Autodesk Inventor part; units mm, degrees
ref_plane "YZ Plane" through (0, 0, 0) normal (1, 0, 0) x (0, 1, 0)
ref_plane "XZ Plane" through (0, 0, 0) normal (0, 1, 0) x (-1, 0, 0)
ref_plane "XY Plane" through (0, 0, 0) normal (0, 0, 1) x (1, 0, 0)
sketch "Sketch1" plane through (0, 0, 0) normal (0, 1, 0) x (-1, 0, 0)
  line L0 (-22, -5) -> (22, -5)
  line L1 (22, 0) -> (22, 0)
  line L2 (22, 5) -> (-22, 5)
  line L3 (-22, 0) -> (-22, 0)
  line L4 (-22, -5) -> (22, 5) construction
  line L5 (22, -5) -> (-22, 5) construction
  circle A0 centre (19.5, 0) radius 1
  line L6 (-22, 5) -> (-22, -5)
  line L7 (22, 5) -> (22, -5)
  circle A1 centre (-19.5, 0) radius 1
  point P0 (0, 0)
  dimension "d0" = 10
  dimension "d1" = 44
  dimension "d3" = 2
  dimension "d6" = 2.5
  dimension "d8" = 5
  dimension "d13" = 2
  dimension "d14" = 2.5
  dimension "d15" = 5
extrude "Extrusion1" add sketch "Sketch1" along normal blind 5
properties part number "link"
Verification items for the finished model (mm, model axes). Give positions to 0.01 mm unless a question says otherwise; leave off trailing zeros. Loops run counter-clockwise (first coordinate to the right, second up) from the corner with the lowest first, then second, coordinate; pieces in that order, holes last. Notation, with made-up numbers: (-9, 23.25) - (19, 23.25) arc R24 cw to (19, 47.25) - close; hole circle Ø6 at (-33.5, 48). An arc over 180 degrees is marked (long way). Write item = value, one per line. Start each with the question number.
Q1. Cross-section at B-B, the plane z = 0. Enter the section's corners in (x, y).
Q2. Mould release check, pull along X, two halves, no side actions. Record for faces 1 (the face through (-18.5, 2.5, 0)), 2 (the face through (0, 2, -5)), 3 (the face through (-22, 2, 0)): released by +X, released by -X, zero draft, split by the parting line, or undercut.
Q3. Cross-section at A-A, the plane x = 19.5. Enter the section's corners in (y, z).
Q4. Thickness scan on line 1 (Z direction, x = 19.5, y = 3); line 2 (X direction, y = 1.4, z = -0.25). Record the ranges inside material, lowest first.
Answer key:
q1.outline = (-22, 0) - (-20.5, 0) - (-20.5, 5) - (-22, 5) - close; (-18.5, 0) - (18.5, 0) - (18.5, 5) - (-18.5, 5) - close; (20.5, 0) - (22, 0) - (22, 5) - (20.5, 5) - close
q2.face_1 = undercut
q2.face_2 = zero draft
q2.face_3 = released by -X
q3.outline = (0, -5) - (5, -5) - (5, -1) - (0, -1) - close; (0, 1) - (5, 1) - (5, 5) - (0, 5) - close
q4.line_1 = -5 to -1, 1 to 5
q4.line_2 = -22 to -20.47, -18.53 to 18.53, 20.47 to 22
